Here's the drawing with two shaded views (mm, measured from the low corner). I have some questions. Round coordinates to 2 decimals unless told otherwise and drop trailing zeros. Loops run counter-clockwise (first coordinate to the right, second up) from the corner with the lowest first, then second, coordinate; pieces in that order, holes last. Notation, with made-up numbers: (2.5, -17) -> (24.5, -17) arc R7 ccw to (24.5, -9) -> close; hole circle Ø5 at (62.25, 66). An arc over 180 degrees is marked (long way). Write item = value, one per line.
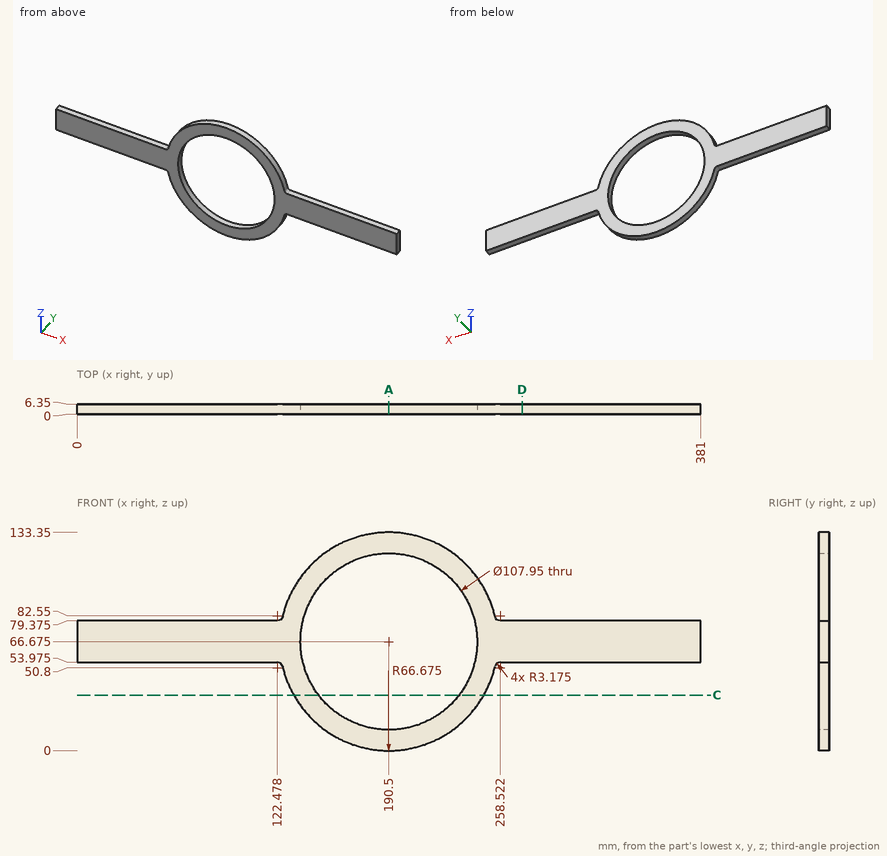
1. Suppose I cut it at D-D, the plane x = 272. List the corners of the cut face in (y, z) for me (3 decimals).
Entries:
outline = (0, 53.975) -> (6.35, 53.975) -> (6.35, 79.375) -> (0, 79.375) -> close
2. Suppose I cut it at A-A, the plane x = 190.5. List the corners of the cut face in (y, z) for me, and give its area (3 significant figures).
Entries:
outline = (0, 0) -> (6.35, 0) -> (6.35, 12.7) -> (0, 12.7) -> close; (0, 120.65) -> (6.35, 120.65) -> (6.35, 133.35) -> (0, 133.35) -> close
area = 161 mm²
3. I'm going to push flat-ended pins straight in: pin 1 (2 mm diameter, centred on x = 160, y = 1.5, fed in from -Z); pin 2 (2 mm diameter, centred on x = 48.5, y = 3, fed in from +Z) (3 decimals); pin 3 (12 mm diameter, centred on x = 159.5, z = 111.5, fed in from -Y); pin 4 (3 mm diameter, centred on x = 136.5, y = 5.5, fed in from -Z). Where does each tip first touch, or does it pass through?
Entries:
pin_1 = 6.88
pin_2 = 79.375
pin_3 = 0
pin_4 = 25.57
4. I need wall thicknesses on line 1 (Z direction, x = 35.5, y = 5) (3 decimals); line 2 (Z direction, x = 191, y = 4); line 3 (X direction, y = 2.5, z = 24). Which ranges of each line are inside material? Lowest first, please. Write a range as [from, to].
Entries:
line_1 = [53.975, 79.375]
line_2 = [0, 12.7], [120.65, 133.35]
line_3 = [139.27, 157.45], [223.55, 241.73]
5. Suppose I cut it at C-C, the plane z = 34. List the corners of the cut face in (x, y) for me.
Entries:
outline = (132.38, 0) -> (147.54, 0) -> (147.54, 6.35) -> (132.38, 6.35) -> close; (233.46, 0) -> (248.62, 0) -> (248.62, 6.35) -> (233.46, 6.35) -> close
